from build123d import *

# Parameters (mm, degrees)
SKETCH1_R           = 1.5
BOSS_EXTRUDE1_DEPTH = 100
SKETCH2_W           = 15
SKETCH2_H           = 0.5
BOSS_EXTRUDE2_DEPTH = 5


with BuildPart() as part:
    # Sketch1 → Boss-Extrude1 (new body, symmetric)
    with BuildSketch(Plane(origin=(0, 0, 0), x_dir=(1, 0, 0), z_dir=(0, 1, 0))):
        Circle(SKETCH1_R)
    extrude(amount=BOSS_EXTRUDE1_DEPTH, both=True)

    # Sketch2 → Boss-Extrude2 (add)
    with BuildSketch(Plane(origin=(0, 100, 0), x_dir=(1, 0, 0), z_dir=(0, 1, 0))):
        Rectangle(SKETCH2_W, SKETCH2_H)
    extrude(amount=-BOSS_EXTRUDE2_DEPTH)


solid = part.part
CAD build for the part. Positions are in the model's coordinates, mm. A direction names the side the tool comes from. Give positions to 0.01 mm unless a question says otherwise; leave off trailing zeros. Loops run counter-clockwise (first coordinate to the right, second up) from the corner with the lowest first, then second, coordinate; pieces in that order, holes last. Notation, with made-up numbers: M 32.25,28.25 L 74.25,28.25 A22 cw 74.25,45.25 Z; hole C -20,32 d6. An arc over 180 degrees is marked long. One line per question, with ' | ' between items. Start each with the question number.
1. Saw through at B-B on x = -4. Give the cut face in (y, z).
2. Saw through at C-C on z = 0.8. Give the cut face in (x, y).
3. Saw through at A-A on y = -61.5. Give the cut face in (x, z).
4. Probe L1, parallel to X at y = -36, z = 0; L2, parallel to Y at x = -1.75, z = 0; L3, parallel to X at y = -79.5, z = -0.85. List the from-to ranges inside material, lowest first. Write a range as from..to.
5. 3-axis set-ups, long thin cutter, end or side, ignore diameter. For faces 1 (the face through (-5, 98, 0.25)), 2 (the face through (-5, 98, -0.25)), 3 (the face through (4, 98, 0.25)), 4 (the face through (4, 98, -0.25)): which of +Z, -Z, +X, -X, +Y, -Y reach the whole face in a straight line?
6. Flat gauge pins, fed straight in: pin 1 (1.5 mm diameter, centred on x = 4, y = 98.5, fed in from +Z); pin 2 (2.5 mm diameter, centred on x = -3.5, y = 96.5, fed in from -Z); pin 3 (0.6 mm diameter, centred on x = -4, z = 0, fed in from -Y). Where does each tip first touch, or does it go through?
Result sheet:
1) outline: M 95,-0.25 L 100,-0.25 L 100,0.25 L 95,0.25 Z
2) outline: M -1.27,-100 L 1.27,-100 L 1.27,100 L -1.27,100 Z
3) outline: C 0,0 d3
4) L1: x = -1.5..1.5 | L2: y = 95..100 | L3: x = -1.24..1.24
5) face 1: +Z, -X, +Y, -Y | face 2: -Z, -X, +Y, -Y | face 3: +Z, +X, +Y, -Y | face 4: -Z, +X, +Y, -Y
6) pin 1: stops at z = 0.25 | pin 2: stops at z = -0.25 | pin 3: stops at y = 95
